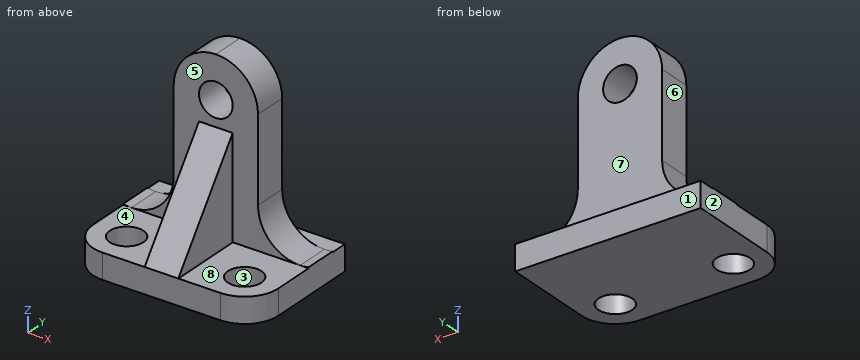
from build123d import *

# Parameters (mm, degrees)
F0_W         = 110
F0_H         = 75
F1_DEPTH     = 115
F2_W         = 10
F2_H         = 100
F3_DEPTH     = 110.001
F4_R         = 10
F5_DEPTH     = 65.001
F6_R         = 10
F7_DEPTH     = 115.001
F9_DEPTH     = 45
F11_DEPTH    = 65.001
F12_T1_DEPTH = 115.5051025722
F12_T3_DEPTH = 115
F14_DEPTH    = 45.0010001
F16_DEPTH    = 45.0010001


# Not quite as in the source:
# - a fillet or chamfer that OpenCascade refuses, or shapes differently, is made with other operations: its cross-section is extruded or revolved along the edge and cut away or added


with BuildPart() as f1:
    # F0 (on Top) → F1 (new body)
    with BuildSketch(Plane.XY):
        with Locations((55, -37.5)):
            Rectangle(F0_W, F0_H)
    extrude(amount=F1_DEPTH)

    # F2 (on face) → F3 (cut, through all)
    with BuildSketch(Plane.YZ.offset(110)):
        with Locations((-5, 65)):
            Rectangle(F2_W, F2_H)
    extrude(amount=-F3_DEPTH, mode=Mode.SUBTRACT)

    # F4 (on face) → F5 (cut, through all)
    with BuildSketch(Plane(origin=(0, -10, 0), x_dir=(-1, 0, 0), z_dir=(0, 1, 0))):
        with BuildLine():
            ThreePointArc((-110, 64.4948974278), (-89.1886116992, 59.364916731), (-80, 40))
            Line((-80, 40), (-80, 90))
            Line((-80, 90), (-80, 115))
            Line((-80, 115), (-110, 115))
            Line((-110, 115), (-110, 64.4948974278))
        make_face()
        with BuildLine():
            ThreePointArc((-105, 15), (-87.3223304703, 22.3223304703), (-80, 40))
            ThreePointArc((-80, 40), (-89.1886116992, 59.364916731), (-110, 64.4948974278))
            Line((-110, 64.4948974278), (-110, 15.5051025722))
            ThreePointArc((-110, 15.5051025722), (-107.5127240501, 15.1265961749), (-105, 15))
        make_face()
        with BuildLine():
            ThreePointArc((0, 64.4948974278), (-20.8113883008, 59.364916731), (-30, 40))
            ThreePointArc((-30, 40), (-22.6776695035, 22.3223304441), (-4.9999999259, 15))
            ThreePointArc((-4.9999999259, 15), (-2.487275913, 15.1265961786), (0, 15.5051025722))
            Line((0, 15.5051025722), (0, 64.4948974278))
        make_face()
        with BuildLine():
            Line((-30, 90), (-30, 40))
            ThreePointArc((-30, 40), (-20.8113883008, 59.364916731), (0, 64.4948974278))
            Line((0, 64.4948974278), (0, 115))
            Line((0, 115), (-30, 115))
            Line((-30, 115), (-30, 90))
        make_face()
        with BuildLine():
            ThreePointArc((-55, 115), (-37.3223304703, 107.6776695297), (-30, 90))
            Line((-30, 90), (-30, 115))
            Line((-30, 115), (-55, 115))
        make_face()
        with BuildLine():
            Line((-80, 115), (-80, 90))
            ThreePointArc((-80, 90), (-72.6776695297, 107.6776695297), (-55, 115))
            Line((-55, 115), (-80, 115))
        make_face()
        with Locations((-55, 90)):
            Circle(F4_R)
    extrude(amount=-F5_DEPTH, mode=Mode.SUBTRACT)

    # F6 (on face) → F7 (cut, through all)
    with BuildSketch(Plane(origin=(0, 0, 0), x_dir=(1, 0, 0), z_dir=(0, 0, -1))):
        with Locations((90, 55)):
            Circle(F6_R)
        with Locations((20, 55)):
            Circle(F6_R)
    extrude(amount=-F7_DEPTH, mode=Mode.SUBTRACT)

    # F8 (on face) → F9 (cut)
    with BuildSketch(Plane.XZ.offset(75)):
        with BuildLine():
            Line((0, 115), (0, 15.5051025722))
            ThreePointArc((0, 15.5051025722), (2.4872759548, 15.1265961744), (5.00000001, 15))
            ThreePointArc((5.00000001, 15), (22.6776695332, 22.3223304739), (30, 40))
            Line((30, 40), (30, 90))
            ThreePointArc((30, 90), (34.0834993366, 103.6930639376), (45, 112.9128784748))
            Line((45, 112.9128784748), (45, 115))
            Line((45, 115), (0, 115))
        make_face()
        with BuildLine():
            ThreePointArc((30, 40), (22.6776695332, 22.3223304739), (5.00000001, 15))
            Line((5.00000001, 15), (45, 15))
            Line((45, 15), (45, 75))
            Line((45, 75), (45, 90))
            Line((45, 90), (45, 112.9128784748))
            ThreePointArc((45, 112.9128784748), (34.0834993366, 103.6930639376), (30, 90))
            Line((30, 90), (30, 40))
        make_face()
        with BuildLine():
            ThreePointArc((105.0000000223, 15), (107.5127240612, 15.126596176), (110, 15.5051025722))
            Line((110, 15.5051025722), (110, 115))
            Line((110, 115), (65, 115))
            Line((65, 115), (65, 112.9128784748))
            ThreePointArc((65, 112.9128784748), (75.9165006634, 103.6930639376), (80, 90))
            Line((80, 90), (80, 40))
            ThreePointArc((80, 40), (87.3223304782, 22.3223304625), (105.0000000223, 15))
        make_face()
        with BuildLine():
            Line((65, 15), (105.0000000223, 15))
            ThreePointArc((105.0000000223, 15), (87.3223304782, 22.3223304625), (80, 40))
            Line((80, 40), (80, 90))
            ThreePointArc((80, 90), (75.9165006634, 103.6930639376), (65, 112.9128784748))
            Line((65, 112.9128784748), (65, 90))
            Line((65, 90), (65, 75))
            Line((65, 75), (65, 15))
        make_face()
        with BuildLine():
            Line((45, 90), (45, 75))
            Line((45, 75), (65, 75))
            Line((65, 75), (65, 90))
            ThreePointArc((65, 90), (55, 80), (45, 90))
        make_face()
        with BuildLine():
            ThreePointArc((65, 112.9128784748), (60.1077410922, 114.4726578233), (55, 115))
            ThreePointArc((55, 115), (49.8922589078, 114.4726578233), (45, 112.9128784748))
            Line((45, 112.9128784748), (45, 90))
            ThreePointArc((45, 90), (55, 100), (65, 90))
            Line((65, 90), (65, 112.9128784748))
        make_face()
        with BuildLine():
            ThreePointArc((65, 90), (55, 100), (45, 90))
            ThreePointArc((45, 90), (55, 80), (65, 90))
        make_face()
    extrude(amount=-F9_DEPTH, mode=Mode.SUBTRACT)

    # F10 (on face) → F11 (cut, through all)
    with BuildSketch(Plane.YZ.offset(65)):
        Polygon((-75, 75), (-75, 15), (-30, 75), align=None)
    extrude(amount=-F11_DEPTH, mode=Mode.SUBTRACT)

    # F12: fillet of radius 20 on 2 edges, made by hand

    # F12_s2 → F12_t1 (cut)
    with BuildSketch(Plane.XY.offset(-50)):
        with BuildLine():
            ThreePointArc((110, -55), (104.1421356237, -69.1421356237), (90, -75))
            Line((90, -75), (110, -75))
            Line((110, -75), (110, -55))
        make_face()
    extrude(amount=F12_T1_DEPTH, mode=Mode.SUBTRACT)

    # F12_s4 → F12_t3 (cut)
    with BuildSketch(Plane.XY.offset(-50)):
        with BuildLine():
            ThreePointArc((20, -75), (5.8578643763, -69.1421356237), (0, -55))
            Line((0, -55), (0, -75))
            Line((0, -75), (20, -75))
        make_face()
    extrude(amount=F12_T3_DEPTH, mode=Mode.SUBTRACT)

    # F14 (cut, through all): a face of the model
    f14_faces = [f1.faces().sort_by_distance(p)[0] for p in [
        (65, -45, 35),
    ]]
    extrude(f14_faces, amount=F14_DEPTH, mode=Mode.SUBTRACT)

    # F15 (on face) → F16 (cut, through all)
    with BuildSketch(Plane(origin=(45, 0, 0), x_dir=(0, -1, 0), z_dir=(-1, 0, 0))):
        Polygon((30, 75), (30, 15), (75, 15), align=None)
    extrude(amount=F16_DEPTH, mode=Mode.SUBTRACT)


solid = f1.part
Design review of the part built by this model. Coordinates are the model's own, in mm. Face numbers are marked on the shaded views. A direction names the side the tool comes from. Round coordinates to 2 decimals unless told otherwise and drop trailing zeros. Loops run counter-clockwise (first coordinate to the right, second up) from the corner with the lowest first, then second, coordinate; pieces in that order, holes last. Notation, with made-up numbers: M 6.5,36 L 32.5,36 A17 cw 32.5,44 Z; hole C 24,-39.5 d11. An arc over 180 degrees is marked long. Answer as a JSON object with one key per item and string values.
Item 1: Clearance check with flat-ended pins moving along their axes: P1, Ø13.5, axis at x = 14.5, y = -61, coming from the +Z side; P2, Ø1.5, axis at y = -15.5, z = 92, coming from the -X side; P3, Ø22.5, axis at y = -60, z = 43.5, coming from the +X side. State where each tip first meets the part, or that it passes through.
Answer sheet:
{"P1": "stops at z = 15", "P2": "stops at x = 30.03", "P3": "stops at x = 65"}
Item 2: We need section B-B on z = 7. Give the boundary of the cut face in (x, y).
Answer sheet:
{"outline": "M 0,-55 A20 ccw 20,-75 L 90,-75 A20 ccw 110,-55 L 110,0 L 0,0 Z; hole C 20,-55 d20; hole C 90,-55 d20"}
Item 3: The part is to be moulded in two halves that separate along X. For the marked faces 1, 2 and 3, say which applies: pulls with the +X half, pulls with the -X half, needs draft (parallel to the pull), parting line crosses it, or undercut.
Answer sheet:
{"face 1": "needs draft", "face 2": "pulls with the -X half", "face 3": "undercut"}
Item 4: We need section C-C on y = -62. Give the boundary of the cut face in (x, z) (3 decimals).
Answer sheet:
{"outline": "M 1.265,0 L 12.859,0 L 12.859,15 L 1.265,15 Z; M 27.141,0 L 82.859,0 L 82.859,15 L 65,15 L 65,32.333 L 45,32.333 L 45,15 L 27.141,15 Z; M 97.141,0 L 108.735,0 L 108.735,15 L 97.141,15 Z"}
Item 5: Machinability: for the marked faces 4, 5, 6, 7 and 8, which of the approach directions +Z, -Z, +X, -X, +Y, -Y give a long, thin tool a straight path to every point of the face, cutting with its end or side? Answer none if there is none.
Answer sheet:
{"face 4": "+Z, -X, -Y", "face 5": "+Z, -Y", "face 6": "+Z, -X, +Y, -Y", "face 7": "+Z, +X, -X, +Y", "face 8": "+Z, +X, -Y"}
Item 6: We need section D-D on z = 92. Give the boundary of the cut face in (x, y), and give its area (3 significant figures).
Answer sheet:
{"outline": "M 30.08,-30 L 45.2,-30 L 45.2,-10 L 30.08,-10 Z; M 64.8,-30 L 79.92,-30 L 79.92,-10 L 64.8,-10 Z", "area": "605 mm^2"}
Item 7: Wall thickness on L1, parallel to X at y = -55, z = 11.5; L2, parallel to Y at x = 90, z = 12; L3, parallel to Z at x = 55, y = -19.5: over which ranges is each line inside the solid? List them lowest first. Write a range as from..to.
Answer sheet:
{"L1": "x = 0..10, 30..80, 100..110", "L2": "y = -75..-65, -45..0", "L3": "z = 0..80, 100..115"}
Item 8: We need section A-A on x = 47. Give the boundary of the cut face in (y, z).
Answer sheet:
{"outline": "M -75,0 L 0,0 L 0,15 L -10,15 L -10,84 L -30,84 L -30,75 L -75,15 Z; M -30,96 L -10,96 L -10,113.69 L -30,113.69 Z"}
